from build123d import *

# Parameters (mm, degrees)
CUT_EXTRUDE1_REACH = 18.637
SKETCH2_R          = 3.175


with BuildPart() as part:
    # Sketch1 → Revolve1 (revolve)
    with BuildSketch(Plane.XY):
        Polygon((-1.5875, -10.4648), (1.5875, -10.4648), (1.5875, -13.2842), (22, -13.4366), (22, -16.637), (-22, -16.637), (-22, -13.4366), (-1.5875, -13.2842), align=None)
    revolve(axis=Axis((-22, 0, 0), (1, 0, 0)))

    # Sketch2 → Cut-Extrude1 (cut, up to next)
    with BuildSketch(Plane.XY, mode=Mode.PRIVATE) as cut_extrude1_sk1:
        with Locations((-18, 0)):
            Circle(SKETCH2_R)
    cut_extrude1_tool1 = extrude(cut_extrude1_sk1.sketch, amount=CUT_EXTRUDE1_REACH, mode=Mode.PRIVATE) & part.part
    add(cut_extrude1_tool1.solids().sort_by_distance((-18, 0, 0))[0], mode=Mode.SUBTRACT)


solid = part.part
Source: CAD feature listing. Evaluate the final solid. Frame: model axes, mm. A direction names the side the tool comes from. Round coordinates to 2 decimals unless told otherwise and drop trailing zeros. Loops run counter-clockwise (first coordinate to the right, second up) from the corner with the lowest first, then second, coordinate; pieces in that order, holes last. Notation, with made-up numbers: (-27.5, 86.5) - (12.5, 86.5) arc R21 ccw to (12.5, 121.5) - close; hole circle Ø6 at (73, 37). An arc over 180 degrees is marked (long way). Write item = value, one per line. Start each with the question number.
Item 1: Mould query, pull axis Y, two halves, no side actions, for faces 4 (the face through (0.022, 2.269, 10.216)), 5 (the face through (-16.293, 2.677, 14.808)), 6 (the face through (-0.308, 2.166, -16.495)), 7 (the face through (22, 1, -14)). Classes: released by +Y, released by -Y, zero draft, split by the parting line, or undercut.
Item 2: Section query C-C on x = 15. Output: boundary loops of the cut face in (y, z).
Item 3: Section query D-D on y = 14.5. Output: boundary loops of the cut face in (x, z), plus the area to 3 significant figures.
Item 4: Section query B-B on y = -1. Count the separate pieces of the cut face and the enclosed holes in it, plus the area to 3 significant figures.
Item 5: Reachability of faces 1 (the face through (-11.651, -7.182, -11.265)), 2 (the face through (11.937, -12.744, -4.013)), 3 (the face through (-22, -1, -14)) from +Z, -Z, +X, -X, +Y, -Y: full face, straight path, thin tool, end or side. Return the list, or none.
Item 6: Section query A-A on x = -9. Output: boundary loops of the cut face in (y, z).
Item 7: Material intervals for line 1 (Z direction, x = 0.25, y = 0); line 2 (X direction, y = 0, z = 14) (3 decimals), sorted ascending.
Item 8: First-contact query: pin 1 Ø12.5 at (y, z) = (0, 0) entering from +X; pin 2 Ø8 at (x, z) = (14, -10.5) entering from +Y; pin 3 Ø13.5 at (y, z) = (6.5, 5.5) entering from +X; pin 4 Ø6 at (x, z) = (7.5, 8) entering from +Y. Flat tips, straight axial feed; report the tip coordinate or a pass-through.
Results list:
q1.face_4 = undercut
q1.face_5 = undercut
q1.face_6 = split by the parting line
q1.face_7 = zero draft
q2.outline = circle Ø33.27 at (0, 0); hole circle Ø26.77 at (0, 0)
q3.outline = (-22, -8.16) - (22, -8.16) - (22, 8.16) - (-22, 8.16) - close
q3.area = 718 mm²
q4.separate_pieces = 3
q4.enclosed_holes = 0
q4.area = 288 mm²
q5.face_1 = -X
q5.face_2 = +X
q5.face_3 = +Z, -Z, -X, +Y, -Y
q6.outline = circle Ø33.27 at (0, 0); hole circle Ø26.68 at (0, 0)
q7.line_1 = -16.64 to -10.46, 10.46 to 16.64
q7.line_2 = -22 to -21.175, -14.825 to 22
q8.pin_1 = through
q8.pin_2 = 15.31
q8.pin_3 = 22
q8.pin_4 = 15.87
